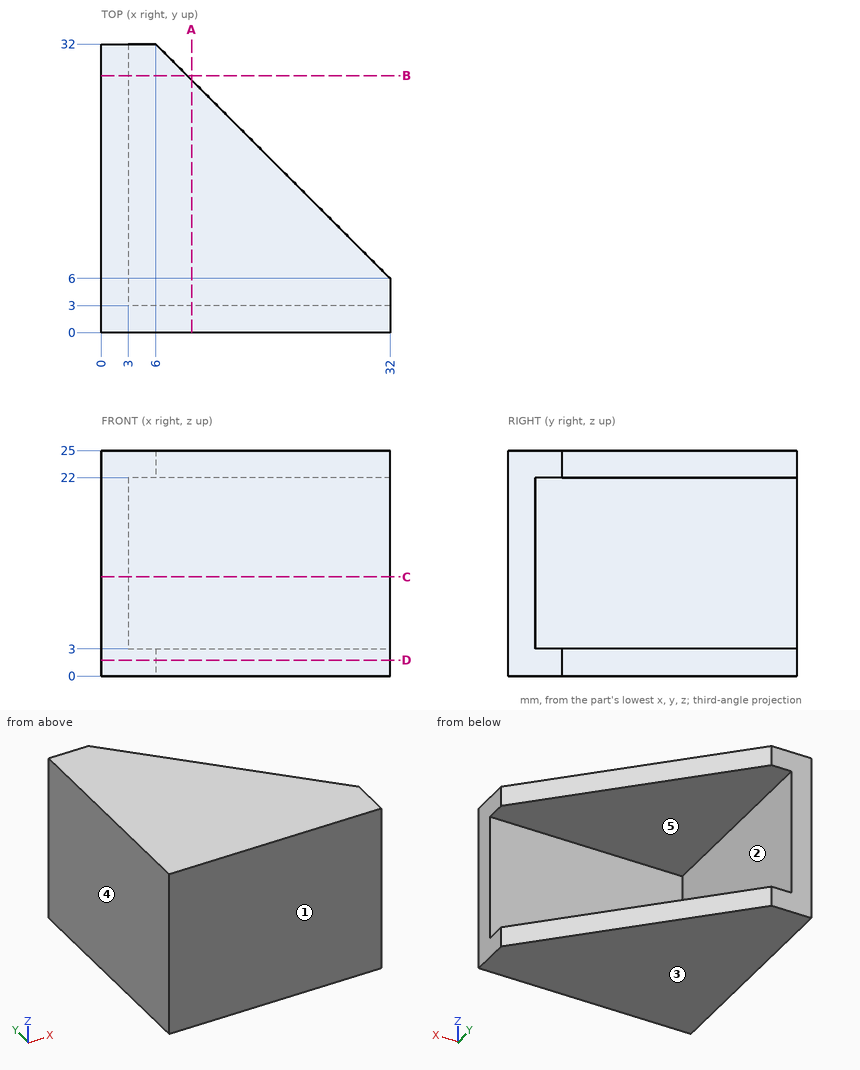
Verification items for this drawing (mm, ordinates from the low corner). A direction names the side the tool comes from. Give positions to 0.01 mm unless a question says otherwise; leave off trailing zeros. Write each loop counter-clockwise with the first axis right and the second up, starting at its lowest first coordinate (ties: lowest second). Pieces come first, ordered by that corner, then holes. Notation, with made-up numbers: (-22.75, -31.5) -> (-14.75, -31.5) arc R16 cw to (-14.75, -26.5) -> close; hole circle Ø2 at (9, 58.5). An arc over 180 degrees is marked (long way). Use CSV: the item, a comma, the result in double quotes.
(1) Sectioned sample at A-A (x = 10). Record the cut outline in (y, z).
Derived:
outline,"(0, 0) -> (28, 0) -> (28, 3) -> (3, 3) -> (3, 22) -> (28, 22) -> (28, 25) -> (0, 25) -> close"
(2) Set-up check for the marked faces 4 and 5: record each of +Z, -Z, +X, -X, +Y, -Y from which the full face is reachable in a straight line by a thin tool's end or side.
Derived:
face 4,"+Z, -Z, -X, +Y, -Y"
face 5,"+X, +Y"
(3) Sectioned sample at C-C (z = 11). Record the cut outline in (x, y), plus the area to 3 significant figures.
Derived:
outline,"(0, 0) -> (32, 0) -> (32, 3) -> (3, 3) -> (3, 32) -> (0, 32) -> close"
area,"183 mm^2"
(4) Go/stop test with flat-tipped pins: pin 1 (4 mm diameter, centred on y = 6, z = 9.5, fed in from +X); pin 2 (5 mm diameter, centred on y = 12, z = 11, fed in from -X); pin 3 (10 mm diameter, centred on x = 12, z = 16, fed in from +Y). Record where each tip stops, or that it passes through.
Derived:
pin 1,"stops at x = 3"
pin 2,"stops at x = 0"
pin 3,"stops at y = 3"
(5) Sectioned sample at B-B (y = 28.5). Record the cut outline in (x, z).
Derived:
outline,"(0, 0) -> (9.5, 0) -> (9.5, 3) -> (3, 3) -> (3, 22) -> (9.5, 22) -> (9.5, 25) -> (0, 25) -> close"
(6) Sectioned sample at D-D (z = 1.75). Record the cut outline in (x, y), plus the area to 3 significant figures.
Derived:
outline,"(0, 0) -> (32, 0) -> (32, 6) -> (6, 32) -> (0, 32) -> close"
area,"686 mm^2"
(7) Material ranges on L1, parallel to Z at x = 9.5, y = 26; L2, parallel to Y at x = 11, z = 13.5, recorded low to high.
Derived:
L1,"z = 0 to 3, 22 to 25"
L2,"y = 0 to 3"
(8) Release check for a two-part mould opening along Z. For the marked faces 1, 2 and 3 record: +Z half, -Z half, draft (parallel to the pull), parting line (faces both ways), or undercut.
Derived:
face 1,"draft"
face 2,"undercut"
face 3,"-Z half"
